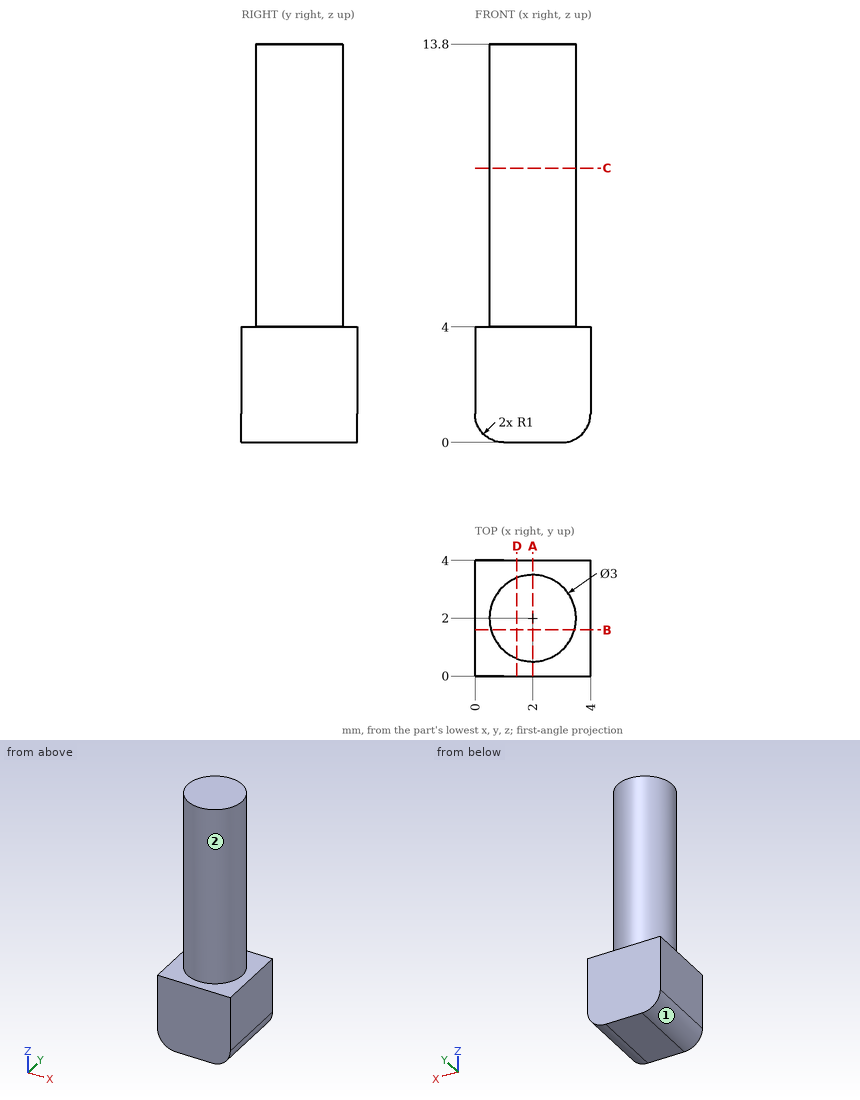
Study the drawing (mm; zero at the part's minimum x, y, z) and answer. A direction names the side the tool comes from. Round coordinates to 2 decimals unless told otherwise and drop trailing zeros. Loops run counter-clockwise (first coordinate to the right, second up) from the corner with the lowest first, then second, coordinate; pieces in that order, holes last.
Q1. Section A-A, the plane x = 2 is taken. Determine the outline of the cut face in (y, z).
Q2. Section C-C, the plane z = 9.5 is taken. Determine the outline of the cut face in (x, y), then the cut area to 3 significant figures.
Q3. Section D-D, the plane x = 1.45 is taken. Determine the outline of the cut face in (y, z), then the cut area to 3 significant figures.
Q4. Given pin 1 Ø1 at (y, z) = (1, 8.5) entering from +X, flat-ended and moving along its own axis, determine where the tip first touches the part or whether it passes through.
Q5. Find the intervals of material crossed by line 1 (Z direction, x = 1.7, y = 0.45); line 2 (Z direction, x = 3.45, y = 0.3); line 3 (Y direction, x = 1.05, z = 10), in increasing order.
Q6. Section B-B, the plane y = 1.6 is taken. Determine the outline of the cut face in (x, z).
Q7. Which of the six approach directions +Z, -Z, +X, -X, +Y, -Y give full straight-line access (tool end or side, diameter ignored) to the marked faces 1 and 2?
Completed:
1. outline: (0, 0) - (4, 0) - (4, 4) - (3.5, 4) - (3.5, 13.8) - (0.5, 13.8) - (0.5, 4) - (0, 4) - close
2. outline: circle Ø3 at (2, 2)
2. area: 7.07 mm2
3. outline: (0, 0) - (4, 0) - (4, 4) - (3.4, 4) - (3.4, 13.8) - (0.6, 13.8) - (0.6, 4) - (0, 4) - close
3. area: 43.4 mm2
4. pin 1: stops at x = 3.41
5. line 1: z = 0 to 4
5. line 2: z = 0.11 to 4
5. line 3: y = 0.84 to 3.16
6. outline: (0, 1) arc R1 ccw to (1, 0) - (3, 0) arc R1 ccw to (4, 1) - (4, 4) - (3.45, 4) - (3.45, 13.8) - (0.55, 13.8) - (0.55, 4) - (0, 4) - close
7. face 1: -Z, -X, +Y, -Y
7. face 2: +Z
